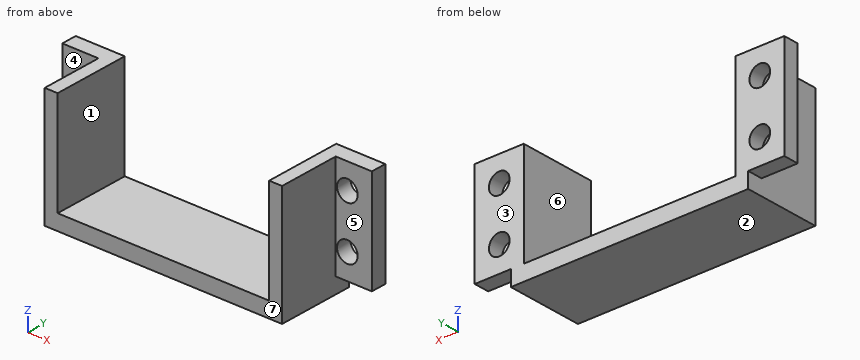
from build123d import *

# Parameters (mm, degrees)
SKETCH1_W           = 46
SKETCH1_H           = 15
BOSS_EXTRUDE1_DEPTH = 3
SKETCH3_W           = 2.5
SKETCH3_H           = 15
BOSS_EXTRUDE2_DEPTH = 20
SKETCH4_W           = 20
SKETCH4_H           = 3
BOSS_EXTRUDE3_DEPTH = 7
SKETCH5_R           = 2
CUT_EXTRUDE1_DEPTH  = 7


with BuildPart() as part:
    # Sketch1 → Boss-Extrude1 (new body)
    with BuildSketch(Plane.XY):
        with Locations((23, 7.5)):
            Rectangle(SKETCH1_W, SKETCH1_H)
    extrude(amount=BOSS_EXTRUDE1_DEPTH)

    # Sketch3 → Boss-Extrude2 (add)
    with BuildSketch(Plane.XY.offset(3)):
        with Locations((1.25, 7.5)):
            Rectangle(SKETCH3_W, SKETCH3_H)
    boss_extrude2 = extrude(amount=BOSS_EXTRUDE2_DEPTH)

    # Sketch4 → Boss-Extrude3 (add)
    with BuildSketch(Plane.ZY):
        with Locations((13, 13.5)):
            Rectangle(SKETCH4_W, SKETCH4_H)
    boss_extrude3 = extrude(amount=BOSS_EXTRUDE3_DEPTH)

    # Sketch5 → Cut-Extrude1 (cut)
    with BuildSketch(Plane(origin=(0, 15, 0), x_dir=(1, 0, 0), z_dir=(0, 1, 0))):
        with Locations(Location((-2.25, -18.1, 0), (0, 0, 270))):
            Circle(SKETCH5_R)
        with Locations(Location((-2.25, -7.9, 0), (0, 0, 270))):
            Circle(SKETCH5_R)
    cut_extrude1 = extrude(amount=-CUT_EXTRUDE1_DEPTH, mode=Mode.SUBTRACT)

    # Mirror1: Boss-Extrude2, Boss-Extrude3, Cut-Extrude1 across plane
    add(boss_extrude2.mirror(Plane(origin=(23, 0, 0), x_dir=(0, 0, 1), z_dir=(1, 0, 0))))
    add(boss_extrude3.mirror(Plane(origin=(23, 0, 0), x_dir=(0, 0, 1), z_dir=(1, 0, 0))))
    add(cut_extrude1.mirror(Plane(origin=(23, 0, 0), x_dir=(0, 0, 1), z_dir=(1, 0, 0))), mode=Mode.SUBTRACT)


solid = part.part
The model under review builds one solid part; all positions refer to its coordinate system, in mm. Face numbers are marked on the shaded views. A direction names the side the tool comes from. Coordinates: 2 decimals unless noted, no trailing zeros. Loops run counter-clockwise (first coordinate to the right, second up) from the corner with the lowest first, then second, coordinate; pieces in that order, holes last.
(1) Draft analysis for pull direction X (two halves, no side actions). For the marked faces 6 and 7, state which applies: +X half, -X half, draft (parallel to the pull), parting line (faces both ways), or undercut.
Determined:
face 6: undercut
face 7: draft
(2) Consider section A-A, the plane z = 12. Give the boundary of the cut face in (x, y), plus the area to 3 significant figures.
Determined:
outline: (-7, 12) - (0, 12) - (0, 0) - (2.5, 0) - (2.5, 15) - (-7, 15) - close; (43.5, 0) - (46, 0) - (46, 12) - (53, 12) - (53, 15) - (43.5, 15) - close
area: 117 mm2
(3) Consider section D-D, the plane x = 48.25. Give the boundary of the cut face in (y, z).
Determined:
outline: (12, 3) - (15, 3) - (15, 5.9) - (12, 5.9) - close; (12, 9.9) - (15, 9.9) - (15, 16.1) - (12, 16.1) - close; (12, 20.1) - (15, 20.1) - (15, 23) - (12, 23) - close
(4) Consider section C-C, the plane y = 1. Give the boundary of the cut face in (x, z), plus the area to 3 significant figures.
Determined:
outline: (0, 0) - (46, 0) - (46, 23) - (43.5, 23) - (43.5, 3) - (2.5, 3) - (2.5, 23) - (0, 23) - close
area: 238 mm2
(5) Wall thickness on L1, parallel to X at y = 14.4, z = 18.1; L2, parallel to Z at x = 48.25, y = 14; L3, parallel to X at y = 6.25, z = 7: over which ranges is each line inside the solid? List them lowest first.
Determined:
L1: x = -7 to -4.25, -0.25 to 2.5, 43.5 to 46.25, 50.25 to 53
L2: z = 3 to 5.9, 9.9 to 16.1, 20.1 to 23
L3: x = 0 to 2.5, 43.5 to 46
(6) Consider section B-B, the plane z = 7.9. Give the boundary of the cut face in (x, y), plus the area to 3 significant figures.
Determined:
outline: (-7, 12) - (-4.25, 12) - (-4.25, 15) - (-7, 15) - close; (-0.25, 12) - (0, 12) - (0, 0) - (2.5, 0) - (2.5, 15) - (-0.25, 15) - close; (43.5, 0) - (46, 0) - (46, 12) - (46.25, 12) - (46.25, 15) - (43.5, 15) - close; (50.25, 12) - (53, 12) - (53, 15) - (50.25, 15) - close
area: 93.0 mm2
(7) Insertion check: P1, Ø5, axis at x = -2.25, z = 18.1, coming from the +Y side; P2, Ø2, axis at x = 51, z = 14, coming from the -Y side; P3, Ø6, axis at x = 20.5, y = 4.5, coming from the +Z side; P4, Ø6, axis at y = 7, z = 5.5, coming from the -X side. Each pin has a flat end and moves straight along its axis. Give the tip position at first contact, or say it passes through.
Determined:
P1: stops at y = 15
P2: stops at y = 12
P3: stops at z = 3
P4: stops at x = 0
(8) Tool access review of the marked faces 1, 2, 3, 4 and 5: name each direction out of +Z, -Z, +X, -X, +Y, -Y from which nothing blocks a thin tool from reaching the whole face with its end or side.
Determined:
face 1: +Z, +Y, -Y
face 2: -Z, +X, -X, +Y, -Y
face 3: +Z, -Z, +X, -X, +Y
face 4: +Z, -Z, -X, -Y
face 5: +Z, -Z, +X, -Y
